Here's the drawing with two shaded views (mm, measured from the low corner). I have some questions. A direction names the side the tool comes from. Round coordinates to 2 decimals unless told otherwise and drop trailing zeros. Order: outer loops, then holes, each group sorted by start corner. A loop starts at its lowest first (then second) coordinate and runs counter-clockwise, first axis right, second up. Notation, with made-up numbers: (-34.5, -5) - (1.5, -5) arc R17 ccw to (1.5, 5) - close; hole circle Ø11 at (65, 66.5). An arc over 180 degrees is marked (long way). Return JSON: item names as keys, results as strings. Group by question number.
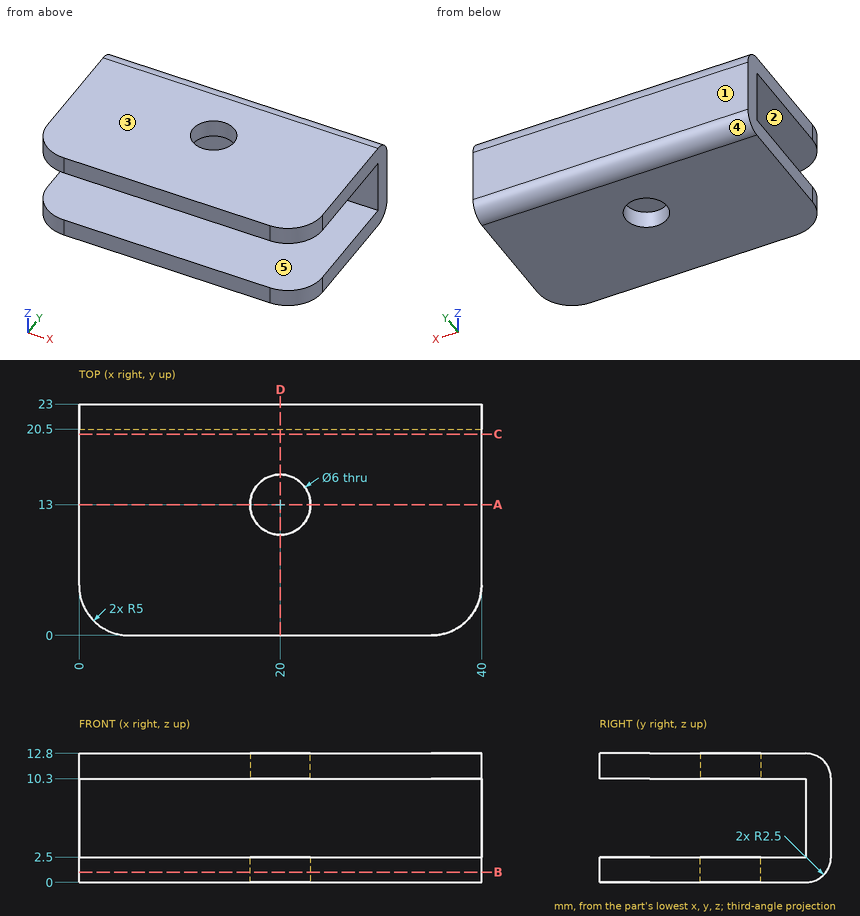
1) I want a section at A-A, the plane y = 13. List the corners of the cut face in (x, z) for me, plus the area to 3 significant figures.
2) I want a section at B-B, the plane z = 1. List the corners of the cut face in (x, y) for me, plus the area to 3 significant figures.
3) I want a section at D-D, the plane x = 20. List the corners of the cut face in (y, z) for me.
4) If I drill on line 1 along Z through (x, y) = (22, 5.75); line 2 along Y through (x, z) = (37, 4); line 3 along X through (y, z) = (12.5, 2.25), over which ranges is the centre line in solid material (lowest first)? Write a range as from..to.
5) Will these pins go through, and if not, where does the flat tip stop? pin 1 (4 mm diameter, centred on x = 20, z = 7.5, fed in from -Y); pin 2 (2 mm diameter, centred on y = 19, z = 9, fed in from -X).
6) We'd pull the mould along Z, two halves only. Please class the marked faces 3, 4 and 5: +Z half, -Z half, draft (parallel to the pull), parting line (faces both ways), or undercut.
7) I want a section at C-C, the plane y = 20. List the corners of the cut face in (x, z) for me.
8) For the marked faces 1 and 2, which set-ups out of +Z, -Z, +X, -X, +Y, -Y let a thin tool reach every point of the face, with its end or its side?
Outcome:
{
 "1": {"outline": "(0, 0) - (17, 0) - (17, 2.5) - (0, 2.5) - close; (0, 10.3) - (17, 10.3) - (17, 12.8) - (0, 12.8) - close; (23, 0) - (40, 0) - (40, 2.5) - (23, 2.5) - close; (23, 10.3) - (40, 10.3) - (40, 12.8) - (23, 12.8) - close", "area": "170 mm^2"},
 "2": {"outline": "(0, 5) arc R5 ccw to (5, 0) - (35, 0) arc R5 ccw to (40, 5) - (40, 22.5) - (0, 22.5) - close; hole circle Ø6 at (20, 13)", "area": "861 mm^2"},
 "3": {"outline": "(0, 0) - (10, 0) - (10, 2.5) - (0, 2.5) - close; (0, 10.3) - (10, 10.3) - (10, 12.8) - (0, 12.8) - close; (16, 0) - (20.5, 0) arc R2.5 ccw to (23, 2.5) - (23, 10.3) arc R2.5 ccw to (20.5, 12.8) - (16, 12.8) - (16, 10.3) - (20.5, 10.3) - (20.5, 2.5) - (16, 2.5) - close"},
 "4": {"line 1": "0..2.5, 10.3..12.8", "line 2": "20.5..23", "line 3": "0..17.04, 22.96..40"},
 "5": {"pin 1": "y = 20.5", "pin 2": "through"},
 "6": {"face 3": "+Z half", "face 4": "-Z half", "face 5": "undercut"},
 "7": {"outline": "(0, 0) - (40, 0) - (40, 2.5) - (0, 2.5) - close; (0, 10.3) - (40, 10.3) - (40, 12.8) - (0, 12.8) - close"},
 "8": {"face 1": "+Z, -Z, +X, -X, +Y", "face 2": "+X, -X, -Y"}
}
